Autodesk Inventor part; units mm, degrees
ref_plane "作業平面4" through (34.5, 0, 0) normal (1, 0, 0) x (0, 0, -1)
ref_plane "作業平面5" through (15.5, 0, 0) normal (1, 0, 0) x (0, 0, -1)
ref_plane "YZ Plane" through (0, 0, 0) normal (1, 0, 0) x (0, 1, 0)
sketch "スケッチ12" plane through (0, 0, 0) normal (1, 0, 0) x (0, 1, 0)
  line L0 (0, 0) -> (-40, 0)
  line L1 (-40, 0) -> (-40, -30)
  line L2 (-40, -30) -> (0, -30)
  line L3 (0, -30) -> (0, 0)
  dimension "d86" = 40
  dimension "d87" = 30
extrude "押し出し15" add sketch "スケッチ12" along normal blind 60
sketch "スケッチ13" plane through (60, 0, 0) normal (1, 0, 0) x (0, 0, -1)
  line L0 (0, 0) -> (0, -2)
  line L1 (2, -10.4) -> (15, -10.4)
  line L2 (15, -10.4) -> (15, -33.6)
  line L3 (15, -33.6) -> (2, -33.6)
  line L4 (2, -33.6) -> (2, -10.4)
  line L5 (30, 0) -> (0, 0)
  line L6 (30, -40) -> (30, 0)
  line L7 (0, 0) -> (0, -40)
  line L8 (0, -40) -> (30, -40)
  line L9 (30, -40) -> (30, 0)
  line L10 (30, 0) -> (0, 0)
  line L11 (0, 0) -> (0, -40)
  line L12 (0, -40) -> (30, -40)
  line L13 (23, -40) -> (23, 0)
  point P0 (-10, 3.6606)
  point P1 (23, 0)
  point P2 (8.5, -27.6)
  dimension "d94" = 23.2
  dimension "d95" = 10.4
  dimension "d99" = 13
  dimension "d130" = 8
  dimension "d137" = 6
  dimension "d138" = 6.5
  dimension "d145" = 15
  dimension "d146" = 2
extrude "押し出し16" cut sketch "スケッチ13" against normal blind 16.4 contours L1 L2 L3 L4
sketch "スケッチ14" plane through (0, -40, -30) normal (0, 0, -1) x (-1, 0, 0)
  line L0 (0, 0) -> (0, 40)
  line L1 (0, 40) -> (-60, 40)
  line L2 (-60, 0) -> (-60, 40)
  line L3 (0, 0) -> (-60, 0)
  circle A0 centre (-30, 20) radius 2.7
  circle A1 centre (-30, 20) radius 4.75
  line L4 (-30, 20) -> (-54, 20)
  line L5 (-30, 20) -> (-6, 20)
  circle A2 centre (-30, 20) radius 6.5
  circle A3 centre (-6, 20) radius 4
  line L6 (-30, 13.5) -> (-30, 26.5)
  circle A4 centre (-54, 20) radius 4
  line L7 (-29.3229, 13.5354) -> (-5.5833, 16.0218)
  line L8 (-5.5833, 23.9782) -> (-29.3229, 26.4646)
  line L9 (-30.6771, 26.4646) -> (-54.4167, 23.9782)
  line L10 (-30.6771, 13.5354) -> (-54.4167, 16.0218)
  circle A5 centre (-54, 20) radius 0.5
  circle A6 centre (-50, 20) radius 0.5
  circle A7 centre (-46, 20) radius 0.5
  circle A8 centre (-42, 20) radius 0.5
  circle A9 centre (-38, 20) radius 0.5
  circle A10 centre (-6, 20) radius 0.5
  circle A11 centre (-10, 20) radius 0.5
  circle A12 centre (-14, 20) radius 0.5
  circle A13 centre (-18, 20) radius 0.5
  circle A14 centre (-22, 20) radius 0.5
  line L11 (44.5, 22.6) -> (44.5, 22.6)
  line L12 (-15.5, 0) -> (-15.5, 0)
  line L13 (-46.2012, 14.0596) -> (-13.7988, 25.9404)
  line L14 (44.5, 0) -> (44.5, 0)
  line L15 (-15.5, 22.6) -> (-15.5, 22.6)
  line L16 (44.5, 22.6) -> (44.5, 22.6)
  line L17 (44.5, 22.6) -> (-15.5, 0)
  line L18 (44.5, 22.6) -> (-15.5, 22.6)
  line L19 (-15.5, 22.6) -> (44.5, 0)
  point P0 (16, 11.6)
  point P1 (-30, 20)
  point P2 (14.5, 11.3)
  dimension "d170" = 5.4
  dimension "d171" = 9.5
  dimension "d172" = 24
  dimension "d173" = 24
  dimension "d174" = 13
  dimension "d175" = 8
  dimension "d176" = 0
  dimension "d177" = 0
  dimension "d178" = 1
  dimension "d179" = 1
  dimension "d180" = 4
  dimension "d181" = 1
  dimension "d182" = 1
  dimension "d183" = 1
  dimension "d184" = 4
  dimension "d185" = 4
  dimension "d186" = 4
  dimension "d187" = 30
  dimension "d188" = 20
extrude "押し出し17" cut sketch "スケッチ14" against normal blind 4 contours A10 | L19 A11 A3 L18 | A3 A11 L5 L19 | L18 A3 | L7 A2 L5 A14 A13 A12 A11 A3 | L5 A11 L19 | A3 L18 L19 A11 L5 A12 A13 A14 A2 L13 L8 | A3 L19 L18 | A11 L5 A3 | A3 L5 A11 | A2 L6 A1 L5 | L5 A3 A11 L19 | L19 A11 | L13 A2 L8 | L19 A11 A3 | L5 A11 A3 | A2 L13 A1 L6 | L5 A1 L13 A2 | A2 L13 A1 L6 | A12 L5 | L5 A12 | L10 L13 A2 | L6 A0 L5 A1 | A1 L13 A0 L6 | L5 A0 L13 A1 | A14 L5 | L5 A14 | L6 A1 L4 A2 | L13 A0 L6 A1 | L13 L10 A4 A6 L4 A7 A8 A9 A2 | A2 L4 A1 L13 | A1 L4 A0 L13 | L6 L5 A0 | A0 L13 L6 | L5 L13 A0 | A2 L4 A9 A8 A7 A6 A4 L9 | L6 A0 L4 A1 | L13 L6 A0 | A13 L5 | L5 A13 | A5 | A4 A6 | A0 L4 L13 | L4 A0 L6 | A9 L4 | L4 A9 | A6 L4 A4 | A4 L4 A6 | A6 L4 A4 | A4 L4 A6 | A8 L4 | L4 A8 | A7 L4 | L4 A7
ref_plane "作業平面3" through (25, 0, 0) normal (1, 0, 0) x (0, 0, -1)
ref_plane "作業平面4" through (34.5, 0, 0) normal (1, 0, 0) x (0, 0, -1)
ref_plane "作業平面5" through (15.5, 0, 0) normal (1, 0, 0) x (0, 0, -1)
sketch "スケッチ15" plane through (34.5, 0, 0) normal (1, 0, 0) x (0, 0, -1)
  line L0 (2, -10.4) -> (15, -10.4)
  line L1 (15, -33.6) -> (2, -33.6)
  line L2 (15, -10.4) -> (15, -33.6)
  line L3 (2, -10.4) -> (15, -10.4)
  line L4 (2, -33.6) -> (2, -10.4)
  point P0 (0, 0)
extrude "押し出し19" cut sketch "スケッチ13" along normal blind 30 from surface at -25.5 contours L5 L13 L8 L7 L0 | L1 L2 L3 L4
extrude "押し出し20" cut sketch "スケッチ13" against normal blind 30 from surface at -44.5 contours L5 L13 L8 L7 L0 | L1 L2 L3 L4
extrude "押し出し21" cut sketch "スケッチ13" against normal blind 16.4 from surface at -25.5 contours L1 L2 L3 L4
sketch "スケッチ16" plane through (15.5, 0, 0) normal (1, 0, 0) x (0, 0, -1)
  line L0 (23, 0) -> (23, -40)
  line L1 (0, -40) -> (23, -40)
  line L2 (0, 0) -> (0, -40)
  line L3 (23, 0) -> (0, 0)
  line L4 (15, -33.6) -> (2, -33.6)
  line L5 (2, -33.6) -> (2, -10.4)
  line L6 (15, -10.4) -> (15, -33.6)
  line L7 (2, -10.4) -> (15, -10.4)
  circle A0 centre (8.5, -27.6) radius 4.9
  dimension "d140" = 6
  dimension "d141" = 6.5
  dimension "d142" = 9.8
extrude "押し出し22" add sketch "スケッチ16" against normal blind 12 contours A0
sketch "スケッチ17" plane through (18.1, -33.6, -2) normal (0, 1, 0) x (1, 0, 0)
  line L0 (2, 10) -> (9, 10)
  line L1 (9, 10) -> (9, 3)
  line L2 (9, 3) -> (2, 3)
  line L3 (2, 3) -> (2, 10)
  line L4 (0, 13) -> (0, 0)
  line L5 (0, 13) -> (16.4, 13)
  point P0 (-18.1, -2)
  dimension "d147" = 7
  dimension "d148" = 7
  dimension "d149" = 2
  dimension "d150" = 3
extrude "押し出し23" cut sketch "スケッチ17" against normal blind 10
extrude "押し出し24" cut sketch "スケッチ14" against normal blind 1.5 from surface at -4 contours L6 L5 A0 | A0 L13 L6 | L5 L13 A0 | L13 L6 A0 | A0 L4 L13 | L4 A0 L6
ref_plane "作業平面7" through (58, -38, -30) normal (0, 0, -1) x (-1, 0, 0)
sketch "スケッチ18" plane through (58, -38, -30) normal (0, 0, -1) x (-1, 0, 0)
  circle A0 centre (27.1663, 23.0232) radius 2.7
  line L0 (51.583, 19.0449) -> (27.8434, 16.5585)
  arc A1 (51.583, 19.0449) -> (51.583, 27.0014) centre (51.1663, 23.0232) ccw
  line L1 (27.8434, 29.4878) -> (51.583, 27.0014)
  arc A2 (27.8434, 29.4878) -> (26.4892, 29.4878) centre (27.1663, 23.0232) ccw
  line L2 (2.7497, 27.0014) -> (26.4892, 29.4878)
  arc A3 (2.7497, 27.0014) -> (2.7497, 19.0449) centre (3.1663, 23.0232) ccw
  line L3 (26.4892, 16.5585) -> (2.7497, 19.0449)
  arc A4 (26.4892, 16.5585) -> (27.8434, 16.5585) centre (27.1663, 23.0232) ccw
  line L4 (3.5833, 21.9782) -> (27.3229, 24.4646)
  line L5 (52.4167, 14.0218) -> (28.6771, 11.5354)
  arc A5 (52.4167, 14.0218) -> (52.4167, 21.9782) centre (52, 18) ccw
  line L6 (28.6771, 24.4646) -> (52.4167, 21.9782)
  arc A6 (28.6771, 24.4646) -> (27.3229, 24.4646) centre (28, 18) ccw
  line L7 (3.5833, 21.9782) -> (27.3229, 24.4646)
  arc A7 (3.5833, 21.9782) -> (3.5833, 14.0218) centre (4, 18) ccw
  line L8 (27.3229, 11.5354) -> (3.5833, 14.0218)
  arc A8 (27.3229, 11.5354) -> (28.6771, 11.5354) centre (28, 18) ccw
  arc A9 (3.5521, 22.2766) -> (3.5521, 13.7234) centre (4, 18) ccw
  line L9 (3.5521, 22.2766) -> (27.2917, 24.763)
  arc A10 (28.7083, 24.763) -> (27.2917, 24.763) centre (28, 18) ccw
  line L10 (28.7083, 24.763) -> (52.4479, 22.2766)
  arc A11 (52.4479, 13.7234) -> (52.4479, 22.2766) centre (52, 18) ccw
  line L11 (52.4479, 13.7234) -> (28.7083, 11.237)
  arc A12 (27.2917, 11.237) -> (28.7083, 11.237) centre (28, 18) ccw
  line L12 (27.2917, 11.237) -> (3.5521, 13.7234)
  point P0 (58, 38)
  dimension "d189" = 0.3
extrude "押し出し25" cut sketch "スケッチ18" against normal blind 4 contours L6 A6 L4 A0 L9 A10 L10 | A0 L10 A11 A1 A5 L6 | L4 A7 A3 A9 L9 A0 | A1 A11 L11 A12 L12 A9 A3 A7 L8 A8 L5 A5
extrude "押し出し26" cut sketch "スケッチ14" against normal blind 2 from surface at -4 contours A11 L5 A3 | A3 L5 A11 | L5 A3 A11 L19 | L19 A11 | L5 A11 A3 | A6 L4 A4 | A4 L4 A6 | A6 L4 A4 | A4 L4 A6 picked at (-9.8359, 20.0907)
ref_plane "作業平面6" through (34.5, -38, 0) normal (1, 0, 0) x (0, 0, -1)
sketch "スケッチ19" plane through (34.5, -38, 0) normal (1, 0, 0) x (0, 0, -1)
  line L0 (2, 4.4) -> (2, 27.6)
  line L1 (2, 27.6) -> (15, 27.6)
  line L2 (15, 27.6) -> (15, 4.4)
  line L3 (15, 4.4) -> (2, 4.4)
  circle A0 centre (8.5, 2.15) radius 1.5
  circle A1 centre (8.5, 29.85) radius 1.5
  point P0 (0, 38)
  dimension "d161" = 3
  dimension "d162" = 3
  dimension "d163" = 2.25
  dimension "d164" = 2.25
  dimension "d165" = 6.5
  dimension "d167" = 6.5
extrude "押し出し27" cut sketch "スケッチ19" against normal blind 4 contours A0 | A1
sketch "スケッチ20" plane through (0, -40, -30) normal (0, 0, -1) x (-1, 0, 0)
  arc A0 (-29.2917, 26.763) -> (-30.7083, 26.763) centre (-30, 20) ccw
  line L0 (-29.2917, 26.763) -> (-5.5521, 24.2766)
  arc A1 (-5.5521, 15.7234) -> (-5.5521, 24.2766) centre (-6, 20) ccw
  line L1 (-5.5521, 15.7234) -> (-29.2917, 13.237)
  arc A2 (-30.7083, 13.237) -> (-29.2917, 13.237) centre (-30, 20) ccw
  line L2 (-30.7083, 13.237) -> (-54.4479, 15.7234)
  arc A3 (-54.4479, 24.2766) -> (-54.4479, 15.7234) centre (-54, 20) ccw
  line L3 (-54.4479, 24.2766) -> (-30.7083, 26.763)
  line L4 (0, 40) -> (-60, 40)
  line L5 (-60, 0) -> (-60, 40)
  line L6 (0, 0) -> (-60, 0)
  line L7 (0, 0) -> (0, 40)
  point P0 (0, 40)
extrude "押し出し28" add sketch "スケッチ20" along normal blind 4
properties part number "joint5_cover"
Work out the finished part from the listing and answer in its coordinate system (mm). A direction names the side the tool comes from. Coordinates: 2 decimals unless noted, no trailing zeros. Loops run counter-clockwise (first coordinate to the right, second up) from the corner with the lowest first, then second, coordinate; pieces in that order, holes last.
1) Consider probe 1 along Y at (x, z) = (33.5, -8.5); probe 2 along Y at (x, z) = (30, -25.45); probe 3 along Z at (x, y) = (27, -32.5). Determine where each line is inside the solid, lowest interval first.
Results:
probe 1: y = -40 to -37.35, -34.35 to -33.6, -10.4 to -9.65, -6.65 to 0
probe 2: y = -40 to -22.7, -17.3 to 0
probe 3: z = -34 to -15, -2 to 0
2) Section D-D (x = 7) is taken. Give the vertices of the cut face in (y, z), plus the area to 3 significant figures.
Results:
outline: (-40, -34) - (-24.43, -34) - (-24.43, -26) - (-15.57, -26) - (-15.57, -34) - (0, -34) - (0, -23) - (-40, -23) - close; circle Ø9.8 at (-27.6, -8.5)
area: 445 mm2
3) Flat-ended cylindrical pins translate along their axes: pin 1 (1.1 mm diameter, centred on x = 50, y = -20, fed in from -Z); pin 2 (3 mm diameter, centred on y = -10.5, z = -17, fed in from -X); pin 3 (7 mm diameter, centred on y = -13, z = -11.5, fed in from +X); pin 4 (12 mm diameter, centred on x = 44, z = -14.5, fed in from +Y). Find the tip coordinate at first contact, or state that the pin passes through.
Results:
pin 1: stops at z = -26
pin 2: stops at x = 15.5
pin 3: stops at x = 34.5
pin 4: passes through
4) For a pull along Z with two mould halves and no side action, classify faces 1 (the flat face through (0, -20, -28)), 2 (the flat face through (24, -37, -5)), 3 (the flat face through (30, -20, -24.5)), 4 (the flat face through (26, -22, -2)) as +Z half, -Z half, draft (parallel to the pull), parting line (faces both ways), or undercut.
Results:
face 1: draft
face 2: undercut
face 3: -Z half
face 4: undercut
5) Section A-A (z = -8.5) is taken. Give the vertices of the cut face in (x, y), plus the area to 3 significant figures.
Results:
outline: (3.5, -32.5) - (15.5, -32.5) - (15.5, -40) - (20.1, -40) - (20.1, -33.6) - (18.1, -33.6) - (18.1, -10.4) - (34.5, -10.4) - (34.5, -9.65) - (30.5, -9.65) - (30.5, -6.65) - (34.5, -6.65) - (34.5, 0) - (15.5, 0) - (15.5, -22.7) - (3.5, -22.7) - close; (27.1, -40) - (34.5, -40) - (34.5, -37.35) - (30.5, -37.35) - (30.5, -34.35) - (34.5, -34.35) - (34.5, -33.6) - (27.1, -33.6) - close
area: 428 mm2
6) Section C-C (y = -27.6) is taken. Give the vertices of the cut face in (x, z).
Results:
outline: (0, -34) - (60, -34) - (60, -23) - (34.5, -23) - (34.5, -15) - (18.1, -15) - (18.1, -2) - (34.5, -2) - (34.5, 0) - (15.5, 0) - (15.5, -3.6) - (3.5, -3.6) - (3.5, -13.4) - (15.5, -13.4) - (15.5, -23) - (0, -23) - close
7) Section B-B (y = -35.85) is taken. Give the vertices of the cut face in (x, z), plus the area to 3 significant figures.
Results:
outline: (0, -34) - (60, -34) - (60, -23) - (34.5, -23) - (34.5, -10) - (30.5, -10) - (30.5, -7) - (34.5, -7) - (34.5, 0) - (15.5, 0) - (15.5, -23) - (0, -23) - close; hole (20.1, -12) - (27.1, -12) - (27.1, -5) - (20.1, -5) - close
area: 1,040 mm2
8) For faces 5 (the flat face through (26, -22, -15)), 6 (the cylindrical face through (58.3, -20.1, -29.9)), 7 (the flat face through (47, -20, -23)), 8 (the flat face through (27.1, -37, -9)), 9 (the flat face through (8, -20, -23)), determine the directions among +Z, -Z, +X, -X, +Y, -Y from which every point of the face is accessible in a straight line to the end or side of a thin tool.
Results:
face 5: +X
face 6: -Z
face 7: +Z, +X, +Y, -Y
face 8: -Y
face 9: -X, +Y, -Y
